Source: CAD feature listing. Evaluate the final solid. Frame: model axes, mm. Face numbers are marked on the shaded views. A direction names the side the tool comes from. Round coordinates to 2 decimals unless told otherwise and drop trailing zeros. Order: outer loops, then holes, each group sorted by start corner. A loop starts at its lowest first (then second) coordinate and runs counter-clockwise, first axis right, second up. Notation, with made-up numbers: M 33.25,-20.5 L 63.25,-20.5 A21 cw 63.25,5.5 Z; hole C 14.25,22 d10. An arc over 180 degrees is marked long. Use one line per item in the form item = value. Start each with the question number.
Q1. Material intervals for probe 1 along X at (y, z) = (0.3, -15); probe 2 along Y at (x, z) = (-3.5, 6.5); probe 3 along Y at (x, z) = (-3, 1), sorted ascending.
Q2. Section A-A (x = 0). Return the cut outline in (y, z), plus the area to 3 significant figures.
Q3. Section C-C (x = 3.5). Return the cut outline in (y, z), plus the area to 3 significant figures.
Q4. Contact query for flat-ended pins moving along their axis: pin 1 (6 mm diameter, centred on x = 13.5, z = 11.5, fed in from -Y); pin 2 (1.5 mm diameter, centred on x = 12, y = 2.5, fed in from +Z); pin 3 (4 mm diameter, centred on x = 1, z = 16, fed in from +Y); pin 4 (0.5 mm diameter, centred on x = 14, y = 0.5, fed in from +Z). Output: stop coordinate, or through.
Q5. Section B-B (y = 11.5). Return the cut outline in (x, z), plus the area to 3 significant figures.
Q6. Section D-D (z = -8). Return the cut outline in (x, y), plus the area to 3 significant figures.
Q7. Reachability of the marked faces 1 and 2 from +Z, -Z, +X, -X, +Y, -Y: full face, straight path, thin tool, end or side. Return the list, or none.
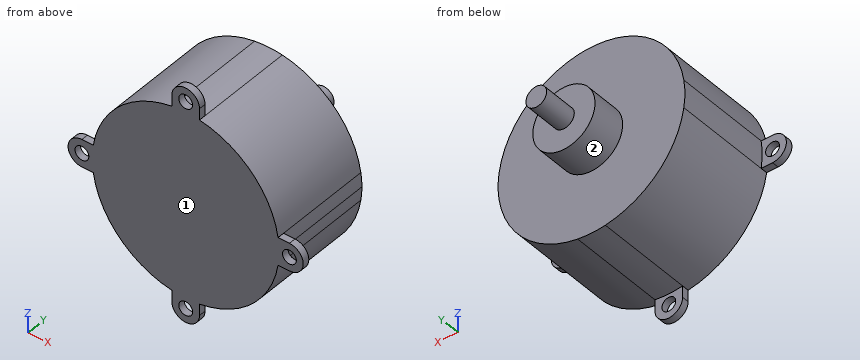
from build123d import *

# Parameters (mm, degrees)
SKETCH1_R           = 1.5
BOSS_EXTRUDE6_DEPTH = 25
SKETCH1_9_R         = 4.5
SKETCH1_9_R_2       = 1.5
BOSS_EXTRUDE7_DEPTH = 20
SKETCH1_10_R        = 4.5
BOSS_EXTRUDE8_DEPTH = 15
SKETCH1_12_R        = 1
BOSS_EXTRUDE9_DEPTH = 1


with BuildPart() as part:
    # Sketch1 → Boss-Extrude6 (new body)
    with BuildSketch(Plane(origin=(0, 0, 0), x_dir=(1, 0, 0), z_dir=(0, 1, 0))):
        with Locations(Location((0, 0, 0), (0, 0, 270))):
            Circle(SKETCH1_R)
    extrude(amount=BOSS_EXTRUDE6_DEPTH)

    # Sketch1_9 → Boss-Extrude7 (add)
    with BuildSketch(Plane(origin=(0, 0, 0), x_dir=(1, 0, 0), z_dir=(0, 1, 0))):
        with Locations(Location((0, 0, 0), (0, 0, 270))):
            Circle(SKETCH1_9_R)
        with Locations(Location((0, 0, 0), (0, 0, 270))):
            Circle(SKETCH1_9_R_2, mode=Mode.SUBTRACT)
    extrude(amount=BOSS_EXTRUDE7_DEPTH)

    # Sketch1_10 → Boss-Extrude8 (add)
    # profile 1 of 5: a face of its own
    with BuildSketch(Plane(origin=(0, 0, 0), x_dir=(1, 0, 0), z_dir=(0, 1, 0))):
        with BuildLine():
            ThreePointArc((13.351029923, 2), (9.545941546, 9.545941546), (2, 13.351029923))
            Line((2, 13.351029923), (2, 11))
            ThreePointArc((2, 11), (4.636038969, 4.636038969), (11, 2))
            Line((11, 2), (13.351029923, 2))
        make_face()
    # profile 2 of 5: a face of its own
    with BuildSketch(Plane(origin=(0, 0, 0), x_dir=(1, 0, 0), z_dir=(0, 1, 0))):
        with BuildLine():
            Line((-2, 11), (-2, 13.351029923))
            ThreePointArc((-2, 13.351029923), (-9.545941546, 9.545941546), (-13.351029923, 2))
            Line((-13.351029923, 2), (-11, 2))
            ThreePointArc((-11, 2), (-4.636038969, 4.636038969), (-2, 11))
        make_face()
    # profile 3 of 5: a face of its own
    with BuildSketch(Plane(origin=(0, 0, 0), x_dir=(1, 0, 0), z_dir=(0, 1, 0))):
        with BuildLine():
            Line((-11, -2), (-13.351029923, -2))
            ThreePointArc((-13.351029923, -2), (-9.545941546, -9.545941546), (-2, -13.351029923))
            Line((-2, -13.351029923), (-2, -11))
            ThreePointArc((-2, -11), (-4.636038969, -4.636038969), (-11, -2))
        make_face()
    # profile 4 of 5: a face of its own
    with BuildSketch(Plane(origin=(0, 0, 0), x_dir=(1, 0, 0), z_dir=(0, 1, 0))):
        with BuildLine():
            Line((2, 11), (2, 13.351029923))
            ThreePointArc((2, 13.351029923), (0, 13.5), (-2, 13.351029923))
            Line((-2, 13.351029923), (-2, 11))
            ThreePointArc((-2, 11), (-4.636038969, 4.636038969), (-11, 2))
            Line((-11, 2), (-13.351029923, 2))
            ThreePointArc((-13.351029923, 2), (-13.5, 0), (-13.351029923, -2))
            Line((-13.351029923, -2), (-11, -2))
            ThreePointArc((-11, -2), (-4.636038969, -4.636038969), (-2, -11))
            Line((-2, -11), (-2, -13.351029923))
            ThreePointArc((-2, -13.351029923), (0, -13.5), (2, -13.351029923))
            Line((2, -13.351029923), (2, -11))
            ThreePointArc((2, -11), (4.636038969, -4.636038969), (11, -2))
            Line((11, -2), (13.351029923, -2))
            ThreePointArc((13.351029923, -2), (13.462705968, -1.002770174), (13.5, 0))
            ThreePointArc((13.5, 0), (13.462705968, 1.002770174), (13.351029923, 2))
            Line((13.351029923, 2), (11, 2))
            ThreePointArc((11, 2), (4.636038969, 4.636038969), (2, 11))
        make_face()
        with Locations(Location((0, 0, 0), (0, 0, 270))):
            Circle(SKETCH1_10_R, mode=Mode.SUBTRACT)
    # profile 5 of 5: a face of its own
    with BuildSketch(Plane(origin=(0, 0, 0), x_dir=(1, 0, 0), z_dir=(0, 1, 0))):
        with BuildLine():
            ThreePointArc((2, -13.351029923), (9.545941546, -9.545941546), (13.351029923, -2))
            Line((13.351029923, -2), (11, -2))
            ThreePointArc((11, -2), (4.636038969, -4.636038969), (2, -11))
            Line((2, -11), (2, -13.351029923))
        make_face()
    extrude(amount=BOSS_EXTRUDE8_DEPTH)

    # Sketch1_12 → Boss-Extrude9 (add)
    # profile 1 of 4: a face of its own
    with BuildSketch(Plane(origin=(0, 0, 0), x_dir=(1, 0, 0), z_dir=(0, 1, 0))):
        with BuildLine():
            ThreePointArc((-13.351029923, -2), (-13.5, 0), (-13.351029923, 2))
            Line((-13.351029923, 2), (-15, 2))
            ThreePointArc((-15, 2), (-17, 0), (-15, -2))
            Line((-15, -2), (-13.351029923, -2))
        make_face()
        with Locations(Location((-15, 0, 0), (0, 0, 270))):
            Circle(SKETCH1_12_R, mode=Mode.SUBTRACT)
    # profile 2 of 4: a face of its own
    with BuildSketch(Plane(origin=(0, 0, 0), x_dir=(1, 0, 0), z_dir=(0, 1, 0))):
        with BuildLine():
            Line((2, -15), (2, -13.351029923))
            ThreePointArc((2, -13.351029923), (0, -13.5), (-2, -13.351029923))
            Line((-2, -13.351029923), (-2, -15))
            ThreePointArc((-2, -15), (0, -17), (2, -15))
        make_face()
        with Locations(Location((0, -15, 0), (0, 0, 270))):
            Circle(SKETCH1_12_R, mode=Mode.SUBTRACT)
    # profile 3 of 4: a face of its own
    with BuildSketch(Plane(origin=(0, 0, 0), x_dir=(1, 0, 0), z_dir=(0, 1, 0))):
        with BuildLine():
            Line((15, 2), (13.351029923, 2))
            ThreePointArc((13.351029923, 2), (13.462705968, 1.002770174), (13.5, 0))
            ThreePointArc((13.5, 0), (13.462705968, -1.002770174), (13.351029923, -2))
            Line((13.351029923, -2), (15, -2))
            ThreePointArc((15, -2), (17, 0), (15, 2))
        make_face()
        with Locations(Location((15, 0, 0), (0, 0, 270))):
            Circle(SKETCH1_12_R, mode=Mode.SUBTRACT)
    # profile 4 of 4: a face of its own
    with BuildSketch(Plane(origin=(0, 0, 0), x_dir=(1, 0, 0), z_dir=(0, 1, 0))):
        with BuildLine():
            Line((2, 13.351029923), (2, 15))
            ThreePointArc((2, 15), (0, 17), (-2, 15))
            Line((-2, 15), (-2, 13.351029923))
            ThreePointArc((-2, 13.351029923), (0, 13.5), (2, 13.351029923))
        make_face()
        with Locations(Location((0, 15, 0), (0, 0, 270))):
            Circle(SKETCH1_12_R, mode=Mode.SUBTRACT)
    extrude(amount=BOSS_EXTRUDE9_DEPTH)


solid = part.part
Results list:
q1.probe_1 = -2 to -1, 1 to 2
q1.probe_2 = 0 to 15
q1.probe_3 = 0 to 20
q2.outline = M 0,-17 L 1,-17 L 1,-16 L 0,-16 Z; M 0,-14 L 1,-14 L 1,-13.5 L 15,-13.5 L 15,-4.5 L 20,-4.5 L 20,-1.5 L 25,-1.5 L 25,1.5 L 20,1.5 L 20,4.5 L 15,4.5 L 15,13.5 L 1,13.5 L 1,14 L 0,14 Z; M 0,16 L 1,16 L 1,17 L 0,17 Z
q2.area = 468 mm2
q3.outline = M 0,-13.04 L 15,-13.04 L 15,-2.83 L 20,-2.83 L 20,2.83 L 15,2.83 L 15,13.04 L 0,13.04 Z
q3.area = 419 mm2
q4.pin_1 = through
q4.pin_2 = 7.46
q4.pin_3 = 1
q4.pin_4 = 2
q5.outline = C 0,0 d27
q5.area = 573 mm2
q6.outline = M -10.87,0 L 10.87,0 L 10.87,15 L -10.87,15 Z
q6.area = 326 mm2
q7.face_1 = +Z, -Z, +X, -X, -Y
q7.face_2 = +Y
